```python
from build123d import *

# Parameters (mm, degrees)
SALIENTE_EXTRUIR1_DEPTH = 5
CROQUIS2_W              = 12
CROQUIS2_H              = 5
SALIENTE_EXTRUIR2_DEPTH = 17
CROQUIS3_R              = 2
CORTAR_EXTRUIR1_DEPTH   = 20
CROQUIS4_R              = 2
CORTAR_EXTRUIR2_DEPTH   = 20


with BuildPart() as part:
    # Croquis1 → Saliente-Extruir1 (new body)
    with BuildSketch(Plane(origin=(0, 0, 0), x_dir=(1, 0, 0), z_dir=(0, 1, 0))):
        Polygon((10.696721311, 25.149180328), (-5.350819672, 25.149180328), (-41.803278689, 25.149180328), (-41.803278689, 20.149180328), (-10.303278689, 20.149180328), (-10.303278689, -25.850819672), (10.696721311, -25.850819672), align=None)
    extrude(amount=SALIENTE_EXTRUIR1_DEPTH)

    # Croquis2 → Saliente-Extruir2 (add)
    with BuildSketch(Plane(origin=(0, 5, 0), x_dir=(1, 0, 0), z_dir=(0, 1, 0))):
        with Locations((-35.803278689, 22.649180328)):
            Rectangle(CROQUIS2_W, CROQUIS2_H)
    extrude(amount=SALIENTE_EXTRUIR2_DEPTH)

    # Croquis3 → Cortar-Extruir1 (cut)
    with BuildSketch(Plane.XZ):
        with Locations(Location((5.696721311, 21.350819672, 0), (0, 0, 270))):
            Circle(CROQUIS3_R)
        with Locations(Location((5.696721311, 11.350819672, 0), (0, 0, 270))):
            Circle(CROQUIS3_R)
        with Locations(Location((5.696721311, 1.350819672, 0), (0, 0, 270))):
            Circle(CROQUIS3_R)
    extrude(amount=-CORTAR_EXTRUIR1_DEPTH, mode=Mode.SUBTRACT)

    # Croquis4 → Cortar-Extruir2 (cut)
    with BuildSketch(Plane.XY.offset(-20.149180328)):
        with Locations((-35.203278689, 16.6)):
            Circle(CROQUIS4_R)
    extrude(amount=-CORTAR_EXTRUIR2_DEPTH, mode=Mode.SUBTRACT)


solid = part.part
```
Work out the finished part from the listing and answer in its coordinate system (mm). A direction names the side the tool comes from. Round coordinates to 2 decimals unless told otherwise and drop trailing zeros. Order: outer loops, then holes, each group sorted by start corner. A loop starts at its lowest first (then second) coordinate and runs counter-clockwise, first axis right, second up.
Q1. A cutting plane is placed at B-B, the plane x = -28. Determine the outline of the cut face in (y, z).
Solution:
outline: (0, -25.15) - (5, -25.15) - (5, -20.15) - (0, -20.15) - close
Q2. A tool of negligible diameter and unlimited length cuts with its end or side. For faces 5 (the flat face through (-10.303, 2, 3)), 6 (the flat face through (-29.803, 13, -23)), 7 (the flat face through (-41.803, 11, -23)), from which of +Z, -Z, +X, -X, +Y, -Y can it reach the whole face along a straight path? Write none if from no direction.
Solution:
face 5: +Z, -X, +Y, -Y
face 6: +Z, -Z, +X, +Y
face 7: +Z, -Z, -X, +Y, -Y
Q3. The mould has two halves that part along Z. Classify faces 1 (the flat face through (-1, 5, 0)), 2 (the cylindrical face through (7.68, 2.46, 1.61)), 3 (the cylindrical face through (5.78, 2.46, 23.35)), 4 (the flat face through (-33, 8, -20.149)): pulls with the +Z half, pulls with the -Z half, needs draft (parallel to the pull), parting line crosses it, or undercut.
Solution:
face 1: needs draft
face 2: undercut
face 3: undercut
face 4: pulls with the +Z half
Q4. A cutting plane is placed at C-C, the plane z = -15.5. Determine the outline of the cut face in (x, y), then the cut area to 3 significant figures.
Solution:
outline: (-10.3, 0) - (10.7, 0) - (10.7, 5) - (-10.3, 5) - close
area: 105 mm2
Q5. Find the intervals of material crossed by line 1 along X through (y, z) = (1.75, -7.5); line 2 along Y through (x, z) = (8.5, -8.5); line 3 along Z through (x, y) = (-32, 17), in increasing order.
Solution:
line 1: x = -10.3 to 10.7
line 2: y = 0 to 5
line 3: z = -25.15 to -20.15
Q6. A cutting plane is placed at A-A, the plane y = 16.6. Determine the outline of the cut face in (x, z), then the cut area to 3 significant figures.
Solution:
outline: (-41.8, -25.15) - (-37.2, -25.15) - (-37.2, -20.15) - (-41.8, -20.15) - close; (-33.2, -25.15) - (-29.8, -25.15) - (-29.8, -20.15) - (-33.2, -20.15) - close
area: 40.0 mm2
Q7. Given pin 1 Ø10 at (x, z) = (-1, -13) entering from +Y; pin 2 Ø2.5 at (y, z) = (2.5, -6) entering from -X; pin 3 Ø3 at (x, y) = (-33.5, 17.5) entering from -Z; pin 4 Ø2.5 at (y, z) = (17.5, -22) entering from +X, each flat-ended and moving along its own axis, determine where each tip first touches the part or whether it passes through.
Solution:
pin 1: stops at y = 5
pin 2: stops at x = -10.3
pin 3: stops at z = -25.15
pin 4: stops at x = -29.8
